Read the model definition and answer for the solid it produces. Units are mm, in the model's axes. Face numbers are marked on the shaded views. A direction names the side the tool comes from. Round coordinates to 2 decimals unless told otherwise and drop trailing zeros. Use a Markdown table: item, result. Add a question column.
1. For the marked faces 1, 2 and 3, determine the directions among +Z, -Z, +X, -X, +Y, -Y from which every point of the face is accessible in a straight line to the end or side of a thin tool.
2. Given pin 1 (3.5 mm diameter, centred on y = -3.5, z = 1, fed in from +X) (3 decimals); pin 2 (6 mm diameter, centred on x = 11, z = -20, fed in from -Y); pin 3 (2 mm diameter, centred on y = -2, z = -1, fed in from +X), each flat-ended and moving along its own axis, determine where each tip first touches the part or whether it passes through.
3. Section A-A, the plane x = 0 is taken. Give the number of separate pieces and of enclosed holes in the cut face, then the cut area to 3 significant figures.
4. The mould has two halves that part along X. Classify the marked faces 4, 5 and 6: +X half, -X half, draft (parallel to the pull), parting line (faces both ways), or undercut.
5. Consider L1, parallel to X at y = -3, z = 1; L2, parallel to X at y = -0.25, z = -13.75 (1 decimal); L3, parallel to Y at x = 9, z = -14.25. Determine where each line is inside the solid, lowest interval first. Write a range as [from, to].
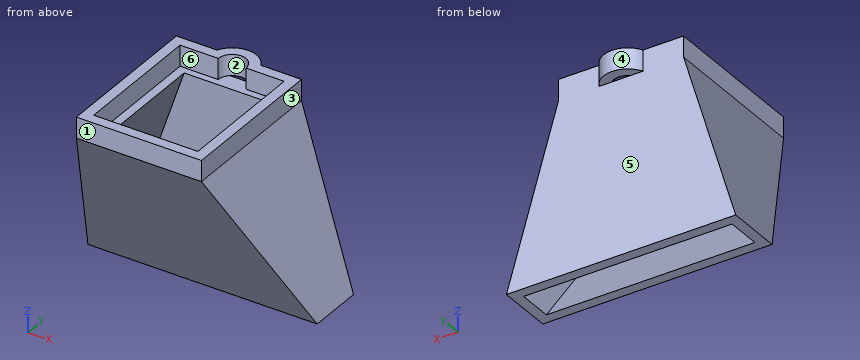
```python
from build123d import *

# Parameters (mm, degrees)
F2_DEPTH = 3
F3_W     = 18
F3_H     = 22
F5_W     = 33
F5_H     = 8
F7_W     = 30
F7_H     = 5
F6_W     = 12.5
F6_H     = 17


with BuildPart() as f2:
    # F1 (on Top) → F2 (new body)
    with BuildSketch(Plane.XY):
        with BuildLine():
            Line((-9, -11), (9, -11))
            Line((9, -11), (9, 11))
            Line((9, 11), (3.1622776602, 11))
            ThreePointArc((3.1622776602, 11), (0, 13), (-3.1622776602, 11))
            Line((-3.1622776602, 11), (-9, 11))
            Line((-9, 11), (-9, -11))
        make_face()
        with BuildLine():
            Line((7.5, 9.5), (7.5, -9.5))
            Line((7.5, -9.5), (-7.5, -9.5))
            Line((-7.5, -9.5), (-7.5, 9.5))
            Line((-7.5, 9.5), (-2, 9.5))
            ThreePointArc((-2, 9.5), (0, 11.5), (2, 9.5))
            Line((2, 9.5), (7.5, 9.5))
        make_face(mode=Mode.SUBTRACT)
    extrude(amount=F2_DEPTH)

    # F3 (on Top) → F8 section 0
    with BuildSketch(Plane.XY):
        Rectangle(F3_W, F3_H)
    # F5 (on offset) → F8 section 1
    with BuildSketch(Plane.XY.offset(-25)):
        with Locations((0, 7)):
            Rectangle(F5_W, F5_H)
    loft()

    # F7 (on face) → F9 section 0
    with BuildSketch(Plane.XY.offset(-25)):
        with Locations((0, 7)):
            Rectangle(F7_W, F7_H)
    # F6 (on face) → F9 section 1
    with BuildSketch(Plane.XY):
        Rectangle(F6_W, F6_H)
    loft(mode=Mode.SUBTRACT)


solid = f2.part
```
Verdict:
| question | item | result |
|---|---|---|
| 1 | face 1 | +Z, -Z, +X, -X, -Y |
| 1 | face 2 | +Z |
| 1 | face 3 | +Z, +X, +Y, -Y |
| 2 | pin 1 | stops at x = 9.225 |
| 2 | pin 2 | stops at y = -1.48 |
| 2 | pin 3 | stops at x = 9.6 |
| 3 | separate pieces | 3 |
| 3 | enclosed holes | 0 |
| 3 | area | 109 mm2 |
| 4 | face 4 | parting line |
| 4 | face 5 | draft |
| 4 | face 6 | undercut |
| 5 | L1 | x = [-9, -7.5], [7.5, 9] |
| 5 | L2 | x = [-13.1, -11.1], [11.1, 13.1] |
| 5 | L3 | y = [-3.02, -1.09], [9.07, 11] |
